```python
from build123d import *

# Parameters (mm, degrees)
SKETCH1_W           = 508
SKETCH1_H           = 23
SKETCH1_R           = 2.5
BOSS_EXTRUDE1_DEPTH = 3.175


with BuildPart() as part:
    # Sketch1 → Boss-Extrude1 (new, symmetric)
    with BuildSketch(Plane(origin=(0, 0, 0), x_dir=(1, 0, 0), z_dir=(0, 1, 0))):
        with Locations((0, 1.5)):
            Rectangle(SKETCH1_W, SKETCH1_H)
        with Locations(Location((-244, 0, 0), (0, 0, 270))):
            Circle(SKETCH1_R, mode=Mode.SUBTRACT)
        with Locations(Location((-189.777777778, 0, 0), (0, 0, 270))):
            Circle(SKETCH1_R, mode=Mode.SUBTRACT)
        with Locations(Location((-135.555555556, 0, 0), (0, 0, 270))):
            Circle(SKETCH1_R, mode=Mode.SUBTRACT)
        with Locations(Location((-81.333333333, 0, 0), (0, 0, 270))):
            Circle(SKETCH1_R, mode=Mode.SUBTRACT)
        with Locations(Location((-27.111111111, 0, 0), (0, 0, 270))):
            Circle(SKETCH1_R, mode=Mode.SUBTRACT)
        with Locations(Location((27.111111111, 0, 0), (0, 0, 270))):
            Circle(SKETCH1_R, mode=Mode.SUBTRACT)
        with Locations(Location((81.333333333, 0, 0), (0, 0, 270))):
            Circle(SKETCH1_R, mode=Mode.SUBTRACT)
        with Locations(Location((135.555555556, 0, 0), (0, 0, 270))):
            Circle(SKETCH1_R, mode=Mode.SUBTRACT)
        with Locations(Location((189.777777778, 0, 0), (0, 0, 270))):
            Circle(SKETCH1_R, mode=Mode.SUBTRACT)
        with Locations(Location((244, 0, 0), (0, 0, 270))):
            Circle(SKETCH1_R, mode=Mode.SUBTRACT)
    extrude(amount=BOSS_EXTRUDE1_DEPTH, both=True)


solid = part.part
```
Check sheet for the modelled part. Datum: model origin and axes. Units: mm. Round coordinates to 2 decimals unless told otherwise and drop trailing zeros. Write item = value, one per line. Start each with the question number.
Q1. Depth check by flat-ended pin: P1, Ø6, axis at x = -27.11, z = 0, coming from the +Y side (3 decimals). Enter the tip coordinate at first touch or a pass-through.
Q2. Section check A-A (y = -0.75). Count the separate pieces of the cut face and the enclosed holes in it, plus the area to 3 significant figures.
Q3. Thickness scan on L1, parallel to Z at x = 244, y = -1.25; L2, parallel to Z at x = 192, y = 2. Record the ranges inside material, lowest first.
Derived:
q1.P1 = 3.175
q2.separate_pieces = 1
q2.enclosed_holes = 10
q2.area = 11,500 mm^2
q3.L1 = -13 to -2.5, 2.5 to 10
q3.L2 = -13 to -1.15, 1.15 to 10
